Build history of the part. All positions in model axes, mm. A direction names the side the tool comes from. Give positions to 0.01 mm unless a question says otherwise; leave off trailing zeros. Write each loop counter-clockwise with the first axis right and the second up, starting at its lowest first coordinate (ties: lowest second). Pieces come first, ordered by that corner, then holes. Notation, with made-up numbers: (41.25, 3) - (48.25, 3) arc R26 ccw to (48.25, 19) - close; hole circle Ø6 at (59.5, 8.25). An arc over 180 degrees is marked (long way). Use one line per item in the form item = value. Start each with the question number.
from build123d import *

# Parameters (mm, degrees)
SKETCH1_R           = 54.6
BOSS_EXTRUDE1_DEPTH = 20
BOSS_EXTRUDE2_DEPTH = 10


with BuildPart() as part:
    # Sketch1 → Boss-Extrude1 (new body)
    with BuildSketch(Plane.XY):
        with BuildLine():
            ThreePointArc((24.815698382, -50.75855705), (16.634074625, -58.135776168), (13.600016394, -68.726187864))
            Line((13.600016394, -68.726187864), (13.600016394, -124.425859017))
            Line((13.600016394, -124.425859017), (-13.600016394, -124.425859017))
            Line((-13.600016394, -124.425859017), (-13.600016394, -68.726187864))
            ThreePointArc((-13.600016394, -68.726187864), (-16.634074625, -58.135776168), (-24.815698382, -50.75855705))
            ThreePointArc((-24.815698382, -50.75855705), (0, 56.5), (24.815698382, -50.75855705))
        make_face()
        Circle(SKETCH1_R, mode=Mode.SUBTRACT)
    extrude(amount=BOSS_EXTRUDE1_DEPTH)

    # Sketch3 → Boss-Extrude2 (add)
    with BuildSketch(Plane(origin=(0, -124.425859017, 0), x_dir=(-1, 0, 0), z_dir=(0, -1, 0))):
        Polygon((4, -16.92820323), (5.615919889, -14.129347882), (0, -10), (-5.615919889, -14.129347882), (-4, -16.92820323), align=None)
        Polygon((-5.615919889, -14.129347882), (0, -10), (-5.615919889, -5.870652118), (-8, -10), align=None)
        Polygon((-5.615919889, -5.870652118), (0, -10), (5.615919889, -5.870652118), (4, -3.07179677), (-4, -3.07179677), align=None)
        Polygon((0, -10), (5.615919889, -14.129347882), (8, -10), (5.615919889, -5.870652118), align=None)
    extrude(amount=BOSS_EXTRUDE2_DEPTH)


solid = part.part
(1) Cut at C-C, the plane y = -32.5. Give the cut face in (x, z), then the cut area to 3 significant figures.
(2) Wall check: line 1 (Y direction, x = 1, z = 14); line 2 (Y direction, x = -3.5, z = 4); line 3 (X direction, y = 10.5, z = 11.25). Give the ranges that are in metal, low to high. Write a range as from..to.
(3) Which spindle directions (+Z, -Z, +X, -X, +Y, -Y) get a long thin tool onto all of the face, cutting with end or side? Do faces 1 (the flat face through (-6, -124.426, 5)), 2 (the flat face through (13.6, -96, 10)), 3 (the flat face through (0, -129, 16.928)), 4 (the flat face through (0, -129, 3.072)). Say none if no direction does.
(4) Cut at D-D, the plane y = -81. Give the cut face in (x, z), then the cut area to 3 significant figures.
(5) Two-plate mould, pull along X, no slides. Class faces 5 (the cylindrical face through (-43.33, -33.22, 9.86)), 6 (the flat face through (-13.6, -97, 10)), 7 (the flat face through (4, -67, 20)): +X half, -X half, draft (parallel to the pull), parting line (faces both ways), or undercut.
(6) Cut at B-B, the plane y = 0. Give the cut face in (x, z).
(7) Cut at A-A, the plane x = 0. Give the cut face in (y, z), then the cut area to 3 significant figures.
(8) Pin check, flat tips, straight feed: pin 1 Ø9 at (x, y) = (-1.5, -129.5) entering from +Z; pin 2 Ø1 at (y, z) = (-105.5, 5) entering from -X; pin 3 Ø1.5 at (x, z) = (9, 9.5) entering from -Y. Stop position of each tip, or through.
Solution:
q1.outline = (-46.22, 0) - (-43.87, 0) - (-43.87, 20) - (-46.22, 20) - close; (43.87, 0) - (46.22, 0) - (46.22, 20) - (43.87, 20) - close
q1.area = 93.7 mm2
q2.line_1 = -134.43..-54.59, 54.59..56.49
q2.line_2 = -134.43..-54.49, 54.49..56.39
q2.line_3 = -55.52..-53.58, 53.58..55.52
q3.face_1 = -Y
q3.face_2 = +Z, -Z, +X, -Y
q3.face_3 = +Z, +X, -X, -Y
q3.face_4 = -Z, +X, -X, -Y
q4.outline = (-13.6, 0) - (13.6, 0) - (13.6, 20) - (-13.6, 20) - close
q4.area = 544 mm2
q5.face_5 = undercut
q5.face_6 = -X half
q5.face_7 = draft
q6.outline = (-56.5, 0) - (-54.6, 0) - (-54.6, 20) - (-56.5, 20) - close; (54.6, 0) - (56.5, 0) - (56.5, 20) - (54.6, 20) - close
q7.outline = (-134.43, 3.07) - (-124.43, 3.07) - (-124.43, 0) - (-54.6, 0) - (-54.6, 20) - (-124.43, 20) - (-124.43, 16.93) - (-134.43, 16.93) - close; (54.6, 0) - (56.5, 0) - (56.5, 20) - (54.6, 20) - close
q7.area = 1,570 mm2
q8.pin_1 = 16.93
q8.pin_2 = -13.6
q8.pin_3 = -124.43
